from build123d import *

# Parameters (mm, degrees)
F1_DEPTH = 25
F0_W     = 62
F0_H     = 23
F2_DEPTH = 3
F4_DEPTH = 25
F5_W     = 21.5
F5_H     = 22
F6_DEPTH = 3
F7_W     = 9
F7_H     = 20
F8_DEPTH = 5
F9_R     = 3


with BuildPart() as f1:
    # F0 (on Top) → F1 (new body)
    with BuildSketch(Plane.XY):
        Polygon((-2.5, 23), (0, 23), (62, 23), (62, 25.5), (-2.5, 25.5), align=None)
        Polygon((0, -2.5), (0, 0), (0, 23), (-2.5, 23), (-2.5, -2.5), align=None)
        Polygon((62, 0), (0, 0), (0, -2.5), (64.5, -2.5), (64.5, 0), align=None)
        Polygon((62, 23), (62, 0), (64.5, 0), (64.5, 25.5), (62, 25.5), align=None)
    extrude(amount=F1_DEPTH)

    # F0 (on Top) → F2 (join)
    with BuildSketch(Plane.XY):
        Polygon((62, 23), (62, 0), (64.5, 0), (64.5, 25.5), (62, 25.5), align=None)
        with Locations((31, 11.5)):
            Rectangle(F0_W, F0_H)
        Polygon((62, 0), (0, 0), (0, -2.5), (64.5, -2.5), (64.5, 0), align=None)
        Polygon((0, -2.5), (0, 0), (0, 23), (-2.5, 23), (-2.5, -2.5), align=None)
        Polygon((-2.5, 23), (0, 23), (62, 23), (62, 25.5), (-2.5, 25.5), align=None)
    extrude(amount=-F2_DEPTH)

    # F3 (on face) → F4 (cut)
    with BuildSketch(Plane(origin=(0, 0, -3), x_dir=(1, 0, 0), z_dir=(0, 0, -1))):
        with BuildLine():
            Line((49, -7.5), (31, -7.5))
            Line((31, -7.5), (13, -7.5))
            ThreePointArc((13, -7.5), (9, -11.5), (13, -15.5))
            Line((13, -15.5), (31, -15.5))
            Line((31, -15.5), (49, -15.5))
            ThreePointArc((49, -15.5), (53, -11.5), (49, -7.5))
        make_face()
    extrude(amount=-F4_DEPTH, mode=Mode.SUBTRACT)

    # F5 (on face) → F6 (cut)
    with BuildSketch(Plane.XZ.offset(2.5)):
        with Locations((16.25, 14)):
            Rectangle(F5_W, F5_H)
        with BuildLine():
            Line((59, 25), (35, 25))
            ThreePointArc((35, 25), (47, 13), (59, 25))
        make_face()
    extrude(amount=-F6_DEPTH, mode=Mode.SUBTRACT)

    # F7 (on face) → F8 (cut)
    with BuildSketch(Plane.YZ.offset(64.5)):
        with Locations((8, 15)):
            Rectangle(F7_W, F7_H)
    extrude(amount=-F8_DEPTH, mode=Mode.SUBTRACT)

    # F9
    f9_edges = [f1.edges().sort_by_distance(p)[0] for p in [
        (64.5, -2.5, 11),
        (64.5, 25.5, 11),
        (-2.5, 25.5, 11),
        (-2.5, -2.5, 11),
    ]]
    fillet(f9_edges, radius=F9_R)


solid = f1.part
Input: part model. Units: mm. Frame: model coordinates. A direction names the side the tool comes from. Give positions to 0.01 mm unless a question says otherwise; leave off trailing zeros. Write each loop counter-clockwise with the first axis right and the second up, starting at its lowest first coordinate (ties: lowest second). Pieces come first, ordered by that corner, then holes. Notation, with made-up numbers: M -28,65.25 L -18,65.25 A19 cw -18,102.25 Z; hole C -16.75,80.5 d1. An arc over 180 degrees is marked long. Write item = value, one per line. Start each with the question number.
1) Cut plane B-B on y = 11.5. Return the cut outline in (x, z), then the cut area to 3 significant figures.
2) Cut plane C-C on z = 8.5. Return the cut outline in (x, y), then the cut area to 3 significant figures.
3) First-contact query: pin 1 Ø1.2 at (y, z) = (-1, 16.5) entering from +X; pin 2 Ø1 at (x, y) = (36.5, 3.5) entering from +Z; pin 3 Ø1.2 at (x, y) = (63, 8.5) entering from +Z. Flat tips, straight axial feed; report the tip coordinate or a pass-through.
4) Material intervals for line 1 along Y through (x, z) = (4, 23); line 2 along X through (y, z) = (22.75, 21); line 3 along X through (y, z) = (-0.25, 23.5), sorted ascending. Write a range as [from, to].
5) Reachability of faces 4 (the flat face through (27, -1, 14)), 5 (the flat face through (63, 8, 5)), 6 (the flat face through (62, 14, 10)), 7 (the flat face through (31, 7.5, -2)) from +Z, -Z, +X, -X, +Y, -Y: full face, straight path, thin tool, end or side. Return the list, or none.
6) Cut plane A-A on x = 17. Return the cut outline in (y, z), then the cut area to 3 significant figures.
7) Cut plane D-D on z = 21. Return the cut outline in (x, y), then the cut area to 3 significant figures.
8) Draft query along X for faces 1 (the flat face through (31, -1, 25)), 2 (the cylindrical face through (-1.6, 24.64, 11.2)), 3 (the flat face through (16, -1, 3)). Return one class per face: +X half, -X half, draft (parallel to the pull), parting line (faces both ways), or undercut.
Solved:
q1.outline = M -2.5,-3 L 9,-3 L 9,0 L 0,0 L 0,25 L -2.5,25 Z; M 53,-3 L 64.5,-3 L 64.5,5 L 62,5 L 62,0 L 53,0 Z
q1.area = 144 mm2
q2.outline = M -2.5,0.5 A3 ccw 0.5,-2.5 L 5.5,-2.5 L 5.5,0 L 0,0 L 0,23 L 62,23 L 62,12.5 L 64.5,12.5 L 64.5,22.5 A3 ccw 61.5,25.5 L 0.5,25.5 A3 ccw -2.5,22.5 Z; M 27,-2.5 L 61.5,-2.5 A3 ccw 64.5,0.5 L 64.5,3.5 L 62,3.5 L 62,0 L 27,0 Z
q2.area = 366 mm2
q3.pin_1 = 64.36
q3.pin_2 = 0
q3.pin_3 = 5
q4.line_1 = [-2.5, 0], [23, 25.5]
q4.line_2 = [-2.49, 0], [62, 64.49]
q4.line_3 = [-2.4, 5.5], [27, 35.09], [58.91, 64.4]
q5.face_4 = +Z, -Y
q5.face_5 = +Z, +X
q5.face_6 = +Z
q5.face_7 = +Z, -Z
q6.outline = M -2.5,-3 L 7.5,-3 L 7.5,0 L 0,0 L 0,3 L -2.5,3 Z; M 15.5,-3 L 25.5,-3 L 25.5,25 L 23,25 L 23,0 L 15.5,0 Z
q6.area = 130 mm2
q7.outline = M -2.5,0.5 A3 ccw 0.5,-2.5 L 5.5,-2.5 L 5.5,0 L 0,0 L 0,23 L 62,23 L 62,12.5 L 64.5,12.5 L 64.5,22.5 A3 ccw 61.5,25.5 L 0.5,25.5 A3 ccw -2.5,22.5 Z; M 27,-2.5 L 35.69,-2.5 L 35.69,0 L 27,0 Z; M 58.31,-2.5 L 61.5,-2.5 A3 ccw 64.5,0.5 L 64.5,3.5 L 62,3.5 L 62,0 L 58.31,0 Z
q7.area = 309 mm2
q8.face_1 = draft
q8.face_2 = -X half
q8.face_3 = undercut
